Could you check a few things on this model? Use its own coordinates, in mm. A direction names the side the tool comes from. Round coordinates to 2 decimals unless told otherwise and drop trailing zeros. Loops run counter-clockwise (first coordinate to the right, second up) from the corner with the lowest first, then second, coordinate; pieces in that order, holes last. Notation, with made-up numbers: (43.5, 46) -> (63.5, 46) arc R15 ccw to (63.5, 51) -> close; hole circle Ø4 at (55, 31.25). An arc over 180 degrees is marked (long way). One line per item, written item: value.
```python
from build123d import *

# Parameters (mm, degrees)
SKETCH_1_R          = 7.5
EXTRUDE_1_DEPTH     = 2
SKETCH_4_R          = 4.5
SKETCH_4_R_2        = 2.85
EXTRUDE_2_DEPTH     = 4.2
SKETCH_5_R          = 2.85
EXTRUDE_3_DEPTH     = 1.7
SKETCH_6_R          = 1.65
CUT_EXTRUDE_1_DEPTH = 13.28576412


with BuildPart() as part:
    # 草图1 → 凸台-拉伸1 (new body)
    with BuildSketch(Plane(origin=(0, 0, 0), x_dir=(1, 0, 0), z_dir=(0, 1, 0))):
        with Locations(Location((0, 0, 0), (0, 0, 270))):
            Circle(SKETCH_1_R)
    extrude(amount=EXTRUDE_1_DEPTH)

    # 草图4 → 凸台-拉伸2 (add)
    with BuildSketch(Plane(origin=(0, 2, 0), x_dir=(1, 0, 0), z_dir=(0, 1, 0))):
        with Locations(Location((0, 0, 0), (0, 0, 270))):
            Circle(SKETCH_4_R)
        with Locations(Location((0, 0, 0), (0, 0, 270))):
            Circle(SKETCH_4_R_2, mode=Mode.SUBTRACT)
    extrude(amount=EXTRUDE_2_DEPTH)

    # 草图5 → 凸台-拉伸3 (add)
    with BuildSketch(Plane(origin=(0, 2, 0), x_dir=(1, 0, 0), z_dir=(0, 1, 0))):
        with Locations(Location((0, 0, 0), (0, 0, 270))):
            Circle(SKETCH_5_R)
    extrude(amount=EXTRUDE_3_DEPTH)

    # 草图6 → 切除-拉伸1 (cut, through all)
    with BuildSketch(Plane.XZ):
        with Locations(Location((0, 0, 0), (0, 0, 270))):
            Circle(SKETCH_6_R)
    extrude(amount=-CUT_EXTRUDE_1_DEPTH, mode=Mode.SUBTRACT)


solid = part.part
```
Item 1: Will this pin go through, and if not, where does the flat tip stop? pin 1 Ø3 at (y, z) = (4.5, -0.5) entering from +X.
Output:
pin 1: stops at x = 4.5
Item 2: If we section it at D-D on x = -2.5: List the corners of the cut face in (y, z) for me.
Output:
outline: (0, -7.07) -> (2, -7.07) -> (2, -3.74) -> (6.2, -3.74) -> (6.2, -1.37) -> (3.7, -1.37) -> (3.7, 1.37) -> (6.2, 1.37) -> (6.2, 3.74) -> (2, 3.74) -> (2, 7.07) -> (0, 7.07) -> close
Item 3: If we mould it in two halves opening along Z, with no side actions, what happens to faces 3 (the face through (1.352, 4.071, 4.292)), 4 (the face through (-5, 2, 0)), 5 (the face through (-1.734, 4.932, -2.262))? For each: released by +Z, released by -Z, zero draft, split by the parting line, or undercut.
Output:
face 3: split by the parting line
face 4: zero draft
face 5: undercut
Item 4: If we section it at C-C on y = 2.25: List the corners of the cut face in (x, z) for me.
Output:
outline: circle Ø9 at (0, 0); hole circle Ø3.3 at (0, 0)
Item 5: If we section it at A-A on z = 0: List the corners of the cut face in (x, y) for me, plus the area to 3 significant figures.
Output:
outline: (-7.5, 0) -> (-1.65, 0) -> (-1.65, 3.7) -> (-2.85, 3.7) -> (-2.85, 6.2) -> (-4.5, 6.2) -> (-4.5, 2) -> (-7.5, 2) -> close; (1.65, 0) -> (7.5, 0) -> (7.5, 2) -> (4.5, 2) -> (4.5, 6.2) -> (2.85, 6.2) -> (2.85, 3.7) -> (1.65, 3.7) -> close
area: 41.3 mm²
Item 6: I need wall thicknesses on line 1 (X direction, y = 4.35, z = 0); line 2 (X direction, y = 2.7, z = 0); line 3 (Y direction, x = -5, z = -4). Which ranges of each line are inside material? Lowest first, please. Write a range as from..to.
Output:
line 1: x = -4.5..-2.85, 2.85..4.5
line 2: x = -4.5..-1.65, 1.65..4.5
line 3: y = 0..2
Item 7: If we section it at B-B on x = 0: List the corners of the cut face in (y, z) for me.
Output:
outline: (0, -7.5) -> (2, -7.5) -> (2, -4.5) -> (6.2, -4.5) -> (6.2, -2.85) -> (3.7, -2.85) -> (3.7, -1.65) -> (0, -1.65) -> close; (0, 1.65) -> (3.7, 1.65) -> (3.7, 2.85) -> (6.2, 2.85) -> (6.2, 4.5) -> (2, 4.5) -> (2, 7.5) -> (0, 7.5) -> close
Item 8: For faces 1 (the face through (-1, 1.82, 1.31)), 2 (the face through (-2, 3.7, 0)), which set-ups out of +Z, -Z, +X, -X, +Y, -Y let a thin tool reach every point of the face, with its end or its side?
Output:
face 1: +Y, -Y
face 2: +Y
